Here's how the part is built. I have some questions about the finished solid (model axes, mm). Face numbers are marked on the shaded views. Coordinates: 2 decimals unless noted, no trailing zeros. Write each loop counter-clockwise with the first axis right and the second up, starting at its lowest first coordinate (ties: lowest second). Pieces come first, ordered by that corner, then holes. Notation, with made-up numbers: (-1, -34.5) -> (35, -34.5) arc R31 cw to (35, -4.5) -> close; hole circle Ø11 at (23, -10.75). An arc over 180 degrees is marked (long way). Use a Markdown table: item, result. Add a question column.
```python
from build123d import *

# Parameters (mm, degrees)
SKETCH_1_W          = 177
SKETCH_1_H          = 65
EXTRUDE_1_DEPTH     = 5
SKETCH_2_W          = 175
SKETCH_2_H          = 2.5
SKETCH_2_H_2        = 55.5
SKETCH_2_H_3        = 0.7
CUT_EXTRUDE_1_DEPTH = 3
FILLET_1_R          = 2
SKETCH_4_W          = 165
SKETCH_4_H          = 6
CUT_EXTRUDE_2_DEPTH = 3


with BuildPart() as part:
    # 草图1 → 凸台-拉伸1 (new body)
    with BuildSketch(Plane.XY):
        Rectangle(SKETCH_1_W, SKETCH_1_H)
    extrude(amount=EXTRUDE_1_DEPTH)

    # 草图2 → 切除-拉伸1 (cut)
    with BuildSketch(Plane.XY.offset(5)):
        with Locations((0, 28.75)):
            Rectangle(SKETCH_2_W, SKETCH_2_H)
        with Locations((0, -2.25)):
            Rectangle(SKETCH_2_W, SKETCH_2_H_2)
        with Locations((0, 30.35)):
            Rectangle(SKETCH_2_W, SKETCH_2_H_3)
    extrude(amount=-CUT_EXTRUDE_1_DEPTH, mode=Mode.SUBTRACT)

    # 圆角1
    fillet_1_edges = [part.edges().sort_by_distance(p)[0] for p in [
        (88.5, -32.5, 2.5),
        (-88.5, -32.5, 2.5),
        (-88.5, 32.5, 2.5),
        (88.5, 32.5, 2.5),
    ]]
    fillet(fillet_1_edges, radius=FILLET_1_R)

    # 草图4 → 切除-拉伸2 (cut)
    with BuildSketch(Plane.XY.offset(2)):
        with Locations((0, 20.5)):
            Rectangle(SKETCH_4_W, SKETCH_4_H)
    extrude(amount=-CUT_EXTRUDE_2_DEPTH, mode=Mode.SUBTRACT)


solid = part.part
```
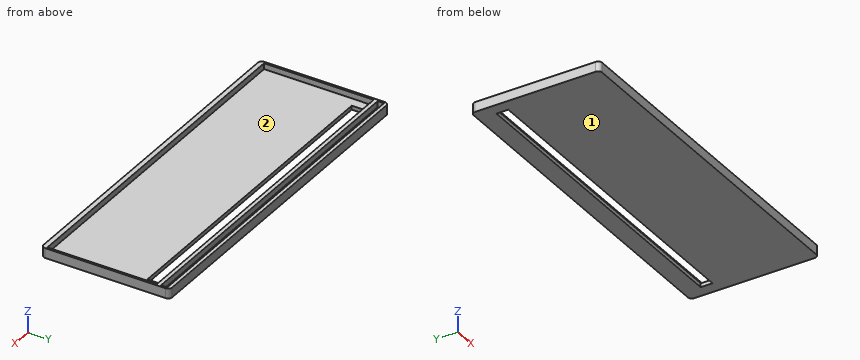
Q1. Suppose I cut it at A-A, the plane y = 21. Write out the boundary of the cut face in (x, z), and give its area (3 significant figures).
Q2. Suppose I cut it at C-C, the plane z = 2.8. Write out the boundary of the cut face in (x, y), and give its area (3 significant figures).
Q3. Thinking about a two-plate mould opening in X: for the marked faces 1 and 2, which applies, released by +X, released by -X, zero draft, split by the parting line, or undercut?
Q4. Will this pin go through, and if not, where does the flat tip stop? pin 1 (8 mm diameter, centred on x = 18.5, y = -25.5, fed in from +Z).
Q5. Suppose I cut it at D-D, the plane y = -18. Write out the boundary of the cut face in (x, z), and give its area (3 significant figures).
Q6. Please list where these lines run through material, in increasing order: line 1 (Y direction, x = 49, z = 4); line 2 (X direction, y = 20.5, z = 2.95); line 3 (Y direction, x = 57, z = 1).
Q7. Suppose I cut it at B-B, the plane x = 43. Write out the boundary of the cut face in (y, z).
Answer key:
| question | item | result |
|---|---|---|
| 1 | outline | (-88.5, 0) -> (-82.5, 0) -> (-82.5, 2) -> (-87.5, 2) -> (-87.5, 5) -> (-88.5, 5) -> close; (82.5, 0) -> (88.5, 0) -> (88.5, 5) -> (87.5, 5) -> (87.5, 2) -> (82.5, 2) -> close |
| 1 | area | 30.0 mm^2 |
| 2 | outline | (-88.5, -30.5) arc R2 ccw to (-86.5, -32.5) -> (86.5, -32.5) arc R2 ccw to (88.5, -30.5) -> (88.5, 30.5) arc R2 ccw to (86.5, 32.5) -> (-86.5, 32.5) arc R2 ccw to (-88.5, 30.5) -> close; hole (-87.5, -30) -> (87.5, -30) -> (87.5, 25.5) -> (-87.5, 25.5) -> close; hole (-87.5, 27.5) -> (87.5, 27.5) -> (87.5, 30.7) -> (-87.5, 30.7) -> close |
| 2 | area | 1,230 mm^2 |
| 3 | face 1 | zero draft |
| 3 | face 2 | undercut |
| 4 | pin 1 | stops at z = 2 |
| 5 | outline | (-88.5, 0) -> (88.5, 0) -> (88.5, 5) -> (87.5, 5) -> (87.5, 2) -> (-87.5, 2) -> (-87.5, 5) -> (-88.5, 5) -> close |
| 5 | area | 360 mm^2 |
| 6 | line 1 | y = -32.5 to -30, 25.5 to 27.5, 30.7 to 32.5 |
| 6 | line 2 | x = -88.5 to -87.5, 87.5 to 88.5 |
| 6 | line 3 | y = -32.5 to 17.5, 23.5 to 32.5 |
| 7 | outline | (-32.5, 0) -> (17.5, 0) -> (17.5, 2) -> (-30, 2) -> (-30, 5) -> (-32.5, 5) -> close; (23.5, 0) -> (32.5, 0) -> (32.5, 5) -> (30.7, 5) -> (30.7, 2) -> (27.5, 2) -> (27.5, 5) -> (25.5, 5) -> (25.5, 2) -> (23.5, 2) -> close |
